Answer from the drawing. Dimensions are ordinates in mm from the lowest x, y and z of the part. A direction names the side the tool comes from. Round coordinates to 2 decimals unless told otherwise and drop trailing zeros. Write each loop counter-clockwise with the first axis right and the second up, starting at its lowest first coordinate (ties: lowest second). Pieces come first, ordered by that corner, then holes. Notation, with made-up numbers: (-36.5, 31.25) - (-11.5, 31.25) arc R24 cw to (-11.5, 60.25) - close; hole circle Ø2 at (10, -25). An arc over 180 degrees is marked (long way). Use a Markdown table: item, result. Add a question column.
1) A cutting plane is placed at C-C (z = 44.5). Give the vertices of the cut face in (x, y) (1 decimal).
2) Each of these flat-tipped pins is pushed along its axis until it touches: P1, Ø1.5, axis at x = 18.5, y = 9.5, coming from the -Z side; P2, Ø1, axis at y = 32.5, z = 25, coming from the -X side; P3, Ø3, axis at x = 6, z = 48, coming from the +Y side. Where does it stop, or does it pass through?
3) A cutting plane is placed at B-B (y = 14.5). Give the vertices of the cut face in (x, z) (1 decimal).
4) A cutting plane is placed at A-A (x = 22). Give the vertices of the cut face in (y, z) (1 decimal), then the cut area to 3 significant figures.
5) A cutting plane is placed at D-D (z = 68). Give the vertices of the cut face in (x, y), then the cut area to 3 significant figures.
6) A tool of negligible diameter and unlimited length cuts with its end or side. For the marked faces 1 and 2, from which of +Z, -Z, +X, -X, +Y, -Y can it reach the whole face along a straight path? Write none if from no direction.
7) Find the intervals of material crossed by probe 1 along Y at (x, z) = (20, 13.5); probe 2 along X at (y, z) = (13.5, 27) (1 decimal), in increasing order. Write a range as from..to.
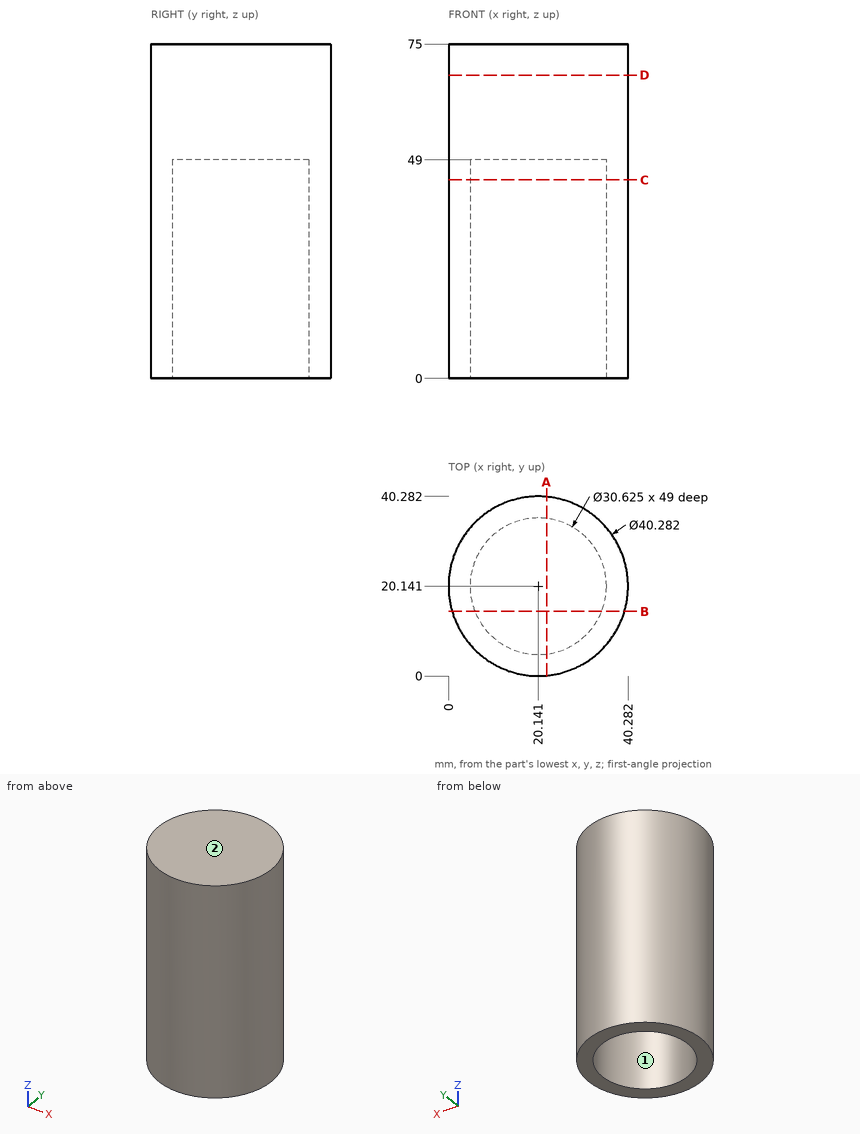
Entries:
| question | item | result |
|---|---|---|
| 1 | outline | circle Ø40.3 at (20.1, 20.1); hole circle Ø30.6 at (20.1, 20.1) |
| 2 | P1 | stops at z = 49 |
| 2 | P2 | stops at x = 3.86 |
| 2 | P3 | stops at y = 35.82 |
| 3 | outline | (0.8, 0) - (5.9, 0) - (5.9, 49) - (34.4, 49) - (34.4, 0) - (39.5, 0) - (39.5, 75) - (0.8, 75) - close |
| 4 | outline | (0.1, 0) - (4.9, 0) - (4.9, 49) - (35.3, 49) - (35.3, 0) - (40.2, 0) - (40.2, 75) - (0.1, 75) - close |
| 4 | area | 1,520 mm² |
| 5 | outline | circle Ø40.28 at (20.14, 20.14) |
| 5 | area | 1,270 mm² |
| 6 | face 1 | -Z |
| 6 | face 2 | +Z, +X, -X, +Y, -Y |
| 7 | probe 1 | y = 0..4.83, 35.45..40.28 |
| 7 | probe 2 | x = 1.1..6.3, 33.9..39.2 |
